```python
from build123d import *

# Parameters (mm, degrees)
PAD_DEPTH    = 2
PAD001_DEPTH = 3


with BuildPart() as part:
    # Sketch → Pad (new body, symmetric)
    with BuildSketch(Plane.XY):
        with BuildLine():
            Line((-7, -4.999991), (-4, 5.000009))
            Line((-4, 5.000009), (-3.799991, 5.000009))
            Line((-3.799991, 5.000009), (-3.799991, 0))
            ThreePointArc((-3.799991, 0), (0, -3.799991), (3.799991, 0))
            Line((3.799991, 5.000009), (3.799991, 0))
            Line((4, 5.000009), (3.799991, 5.000009))
            Line((4, 5.000009), (7, -4.999991))
            Line((7, -4.999991), (-7, -4.999991))
        make_face()
    extrude(amount=PAD_DEPTH, both=True)

    # Sketch004 (on Face10 of Pad) → Pad001 (join)
    with BuildSketch(Plane.XY.offset(2)):
        with BuildLine():
            ThreePointArc((-2.5, 0), (0, -2.5), (2.5, 0))
            Line((2.5, 5.000009), (2.5, 0))
            Line((4, 5.000009), (2.5, 5.000009))
            Line((4, 5.000009), (7, -4.999991))
            Line((7, -4.999991), (-7, -4.999991))
            Line((-7, -4.999991), (-4, 5.000009))
            Line((-4, 5.000009), (-2.5, 5.000009))
            Line((-2.5, 5.000009), (-2.5, 0))
        make_face()
    pad001 = extrude(amount=PAD001_DEPTH)

    # Mirrored: Pad001 across XY
    add(pad001.mirror(Plane.XY))


with BuildPart() as part_1:
    # Body placement: moved
    add(part.part.moved(Location((-23, 0, 0))))


solid = part_1.part
```
For this review, take the finished solid that the model builds, in its own axes (mm). A direction names the side the tool comes from. Round coordinates to 2 decimals unless told otherwise and drop trailing zeros. Write each loop counter-clockwise with the first axis right and the second up, starting at its lowest first coordinate (ties: lowest second). Pieces come first, ordered by that corner, then holes. Notation, with made-up numbers: (0, 52) -> (4, 52) arc R24 ccw to (4, 83) -> close; hole circle Ø6 at (26.25, -8.75). An arc over 180 degrees is marked (long way). Use one line per item in the form item = value.
1) Take a section at D-D, the plane y = -1.25. Write out the cut boundary in (x, z) (3 decimals).
Found:
outline = (-28.875, -5) -> (-25.165, -5) -> (-25.165, -2) -> (-26.589, -2) -> (-26.589, 2) -> (-25.165, 2) -> (-25.165, 5) -> (-28.875, 5) -> close; (-20.835, -5) -> (-17.125, -5) -> (-17.125, 5) -> (-20.835, 5) -> (-20.835, 2) -> (-19.411, 2) -> (-19.411, -2) -> (-20.835, -2) -> close
2) Take a section at B-B, the plane x = -23. Write out the cut boundary in (y, z).
Found:
outline = (-5, -5) -> (-2.5, -5) -> (-2.5, -2) -> (-3.8, -2) -> (-3.8, 2) -> (-2.5, 2) -> (-2.5, 5) -> (-5, 5) -> close
3) Take a section at A-A, the plane y = 1. Write out the cut boundary in (x, z).
Found:
outline = (-28.2, -5) -> (-25.5, -5) -> (-25.5, -2) -> (-26.8, -2) -> (-26.8, 2) -> (-25.5, 2) -> (-25.5, 5) -> (-28.2, 5) -> close; (-20.5, -5) -> (-17.8, -5) -> (-17.8, 5) -> (-20.5, 5) -> (-20.5, 2) -> (-19.2, 2) -> (-19.2, -2) -> (-20.5, -2) -> close
4) Tool access review of faces 1 (the flat face through (-25.5, 3, 3)), 2 (the flat face through (-19.7, 5, 2.3)), 3 (the flat face through (-19.2, 3, 0)): name each direction out of +Z, -Z, +X, -X, +Y, -Y from which nothing blocks a thin tool from reaching the whole face with its end or side.
Found:
face_1 = +Z, -Z, +Y
face_2 = +Z, -Z, +X, -X, +Y
face_3 = +Y
5) Mouldability with a two-part tool opening along X and no side actions: class faces 4 (the cylindrical face through (-23.1, -2.5, -3.5)), 5 (the flat face through (-17.52, 0.07, 0.07)), 6 (the flat face through (-23, -5, 0)) as +X half, -X half, draft (parallel to the pull), parting line (faces both ways), or undercut.
Found:
face_4 = undercut
face_5 = +X half
face_6 = draft
6) To check wall thickness, follow L1, parallel to Z at x = -20.25, y = 1.5; L2, parallel to X at y = 1.5, z = -2.5; L3, parallel to X at y = -3, z = 1.5. State the ranges of each line that lie inside material, in increasing order. Write a range as from..to.
Found:
L1 = -5..-2, 2..5
L2 = -28.05..-25.5, -20.5..-17.95
L3 = -29.4..-25.33, -20.67..-16.6
7) Take a section at C-C, the plane z = -2.75. Write out the cut boundary in (x, y), and give its area (3 significant figures).
Found:
outline = (-30, -5) -> (-16, -5) -> (-19, 5) -> (-20.5, 5) -> (-20.5, 0) arc R2.5 cw to (-25.5, 0) -> (-25.5, 5) -> (-27, 5) -> close
area = 75.2 mm2
8) Clearance check with flat-ended pins moving along their axes: pin 1 (1.5 mm diameter, centred on y = 3, z = 3.5, fed in from -X) (3 decimals); pin 2 (3 mm diameter, centred on y = 3, z = 3, fed in from -X); pin 3 (4 mm diameter, centred on y = 0.5, z = -3.5, fed in from -X). State where each tip first meets the part, or that it passes through.
Found:
pin_1 = -27.825
pin_2 = -28.05
pin_3 = -28.95
